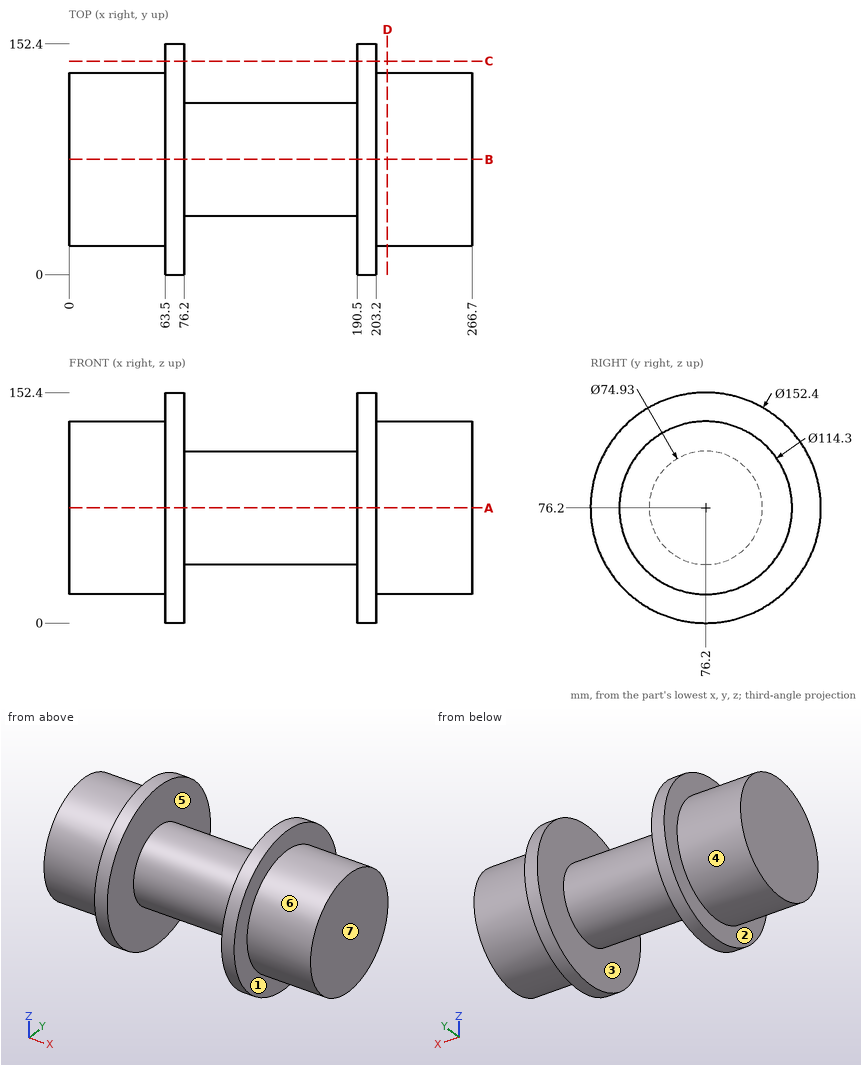
The figure shows three views and two pictorial views of one solid part (mm, origin at its lowest corner). Answer the questions. A direction names the side the tool comes from. Coordinates: 2 decimals unless noted, no trailing zeros. Loops run counter-clockwise (first coordinate to the right, second up) from the corner with the lowest first, then second, coordinate; pieces in that order, holes last.
1) Flat-ended cylindrical pins translate along their axes: pin 1 Ø6 at (x, z) = (142.5, 60) entering from +Y; pin 2 Ø5 at (x, y) = (95, 60) entering from +Z; pin 3 Ø8 at (x, z) = (74, 16) entering from -Y. Find the tip coordinate at first contact, or state that the pin passes through.
2) Find section C-C on y = 141. Write down the section's boundary in (x, z).
3) Find section A-A on z = 76.2. Write down the section's boundary in (x, y) (3 decimals), then the cut area to 3 significant figures.
4) Determine the mould class of the marked faces 1, 2, 3 and 4 for opening direction X: pulls with the +X half, pulls with the -X half, needs draft (parallel to the pull), parting line crosses it, or undercut.
5) Find the intervals of material crossed by L1, parallel to X at y = 54.5, z = 115; L2, parallel to X at y = 62.5, z = 137.5; L3, parallel to Y at x = 195, z = 146, in increasing order.
6) A tool of negligible diameter and unlimited length cuts with its end or side. For the marked faces 5, 6 and 7, from which of +Z, -Z, +X, -X, +Y, -Y can it reach the whole face along a straight path? Write none if from no direction.
7) Find section D-D on x = 210.5. Write down the section's boundary in (y, z), then the cut area to 3 significant figures.
Values:
1. pin 1: stops at y = 111.26
1. pin 2: stops at z = 111.07
1. pin 3: stops at y = 24.74
2. outline: (63.5, 36.11) - (76.2, 36.11) - (76.2, 116.29) - (63.5, 116.29) - close; (190.5, 36.11) - (203.2, 36.11) - (203.2, 116.29) - (190.5, 116.29) - close
3. outline: (0, 19.05) - (63.5, 19.05) - (63.5, 0) - (76.2, 0) - (76.2, 38.735) - (190.5, 38.735) - (190.5, 0) - (203.2, 0) - (203.2, 19.05) - (266.7, 19.05) - (266.7, 133.35) - (203.2, 133.35) - (203.2, 152.4) - (190.5, 152.4) - (190.5, 113.665) - (76.2, 113.665) - (76.2, 152.4) - (63.5, 152.4) - (63.5, 133.35) - (0, 133.35) - close
3. area: 27,000 mm2
4. face 1: pulls with the +X half
4. face 2: pulls with the -X half
4. face 3: undercut
4. face 4: needs draft
5. L1: x = 0 to 76.2, 190.5 to 266.7
5. L2: x = 63.5 to 76.2, 190.5 to 203.2
5. L3: y = 45.63 to 106.77
6. face 5: none
6. face 6: +X
6. face 7: +Z, -Z, +X, +Y, -Y
7. outline: circle Ø114.3 at (76.2, 76.2)
7. area: 10,300 mm2
